Study the drawing (mm; zero at the part's minimum x, y, z) and answer. A direction names the side the tool comes from. Round coordinates to 2 decimals unless told otherwise and drop trailing zeros. Write each loop counter-clockwise with the first axis right and the second up, starting at its lowest first coordinate (ties: lowest second). Pieces come first, ordered by that corner, then holes.
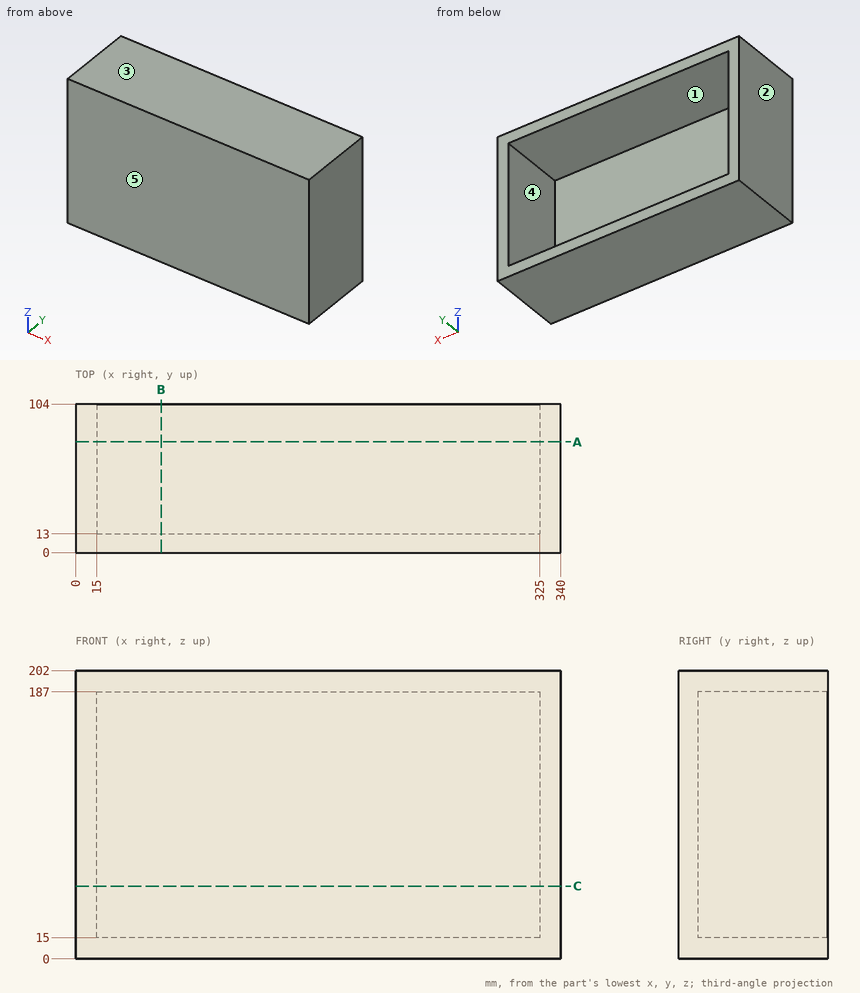
1. A tool of negligible diameter and unlimited length cuts with its end or side. For the marked faces 4 and 5, from which of +Z, -Z, +X, -X, +Y, -Y can it reach the whole face along a straight path? Write none if from no direction.
Geometry says:
face 4: +Y
face 5: +Z, -Z, +X, -X, -Y
2. Section B-B on x = 60 is taken. Determine the outline of the cut face in (y, z).
Geometry says:
outline: (0, 0) - (104, 0) - (104, 15) - (13, 15) - (13, 187) - (104, 187) - (104, 202) - (0, 202) - close
3. Section A-A on y = 77.5 is taken. Determine the outline of the cut face in (x, z).
Geometry says:
outline: (0, 0) - (340, 0) - (340, 202) - (0, 202) - close; hole (15, 15) - (325, 15) - (325, 187) - (15, 187) - close
4. Straight lines are drawn through the part: line 1 along Z through (x, y) = (79.5, 59.5); line 2 along X through (y, z) = (47, 57); line 3 along Y through (x, z) = (143.5, 66). For each, find the intervals that lie inside material, in ascending order.
Geometry says:
line 1: z = 0 to 15, 187 to 202
line 2: x = 0 to 15, 325 to 340
line 3: y = 0 to 13
5. Section C-C on z = 51 is taken. Determine the outline of the cut face in (x, y).
Geometry says:
outline: (0, 0) - (340, 0) - (340, 104) - (325, 104) - (325, 13) - (15, 13) - (15, 104) - (0, 104) - close
6. Given pin 1 (3 mm diameter, centred on x = 195.5, z = 91.5, fed in from -Y); pin 2 (8 mm diameter, centred on x = 211, z = 154, fed in from +Y), each flat-ended and moving along its own axis, determine where each tip first touches the part or whether it passes through.
Geometry says:
pin 1: stops at y = 0
pin 2: stops at y = 13
7. For a pull along X with two mould halves and no side action, classify the marked faces 1, 2 and 3 as released by +X, released by -X, zero draft, split by the parting line, or undercut.
Geometry says:
face 1: undercut
face 2: released by -X
face 3: zero draft
